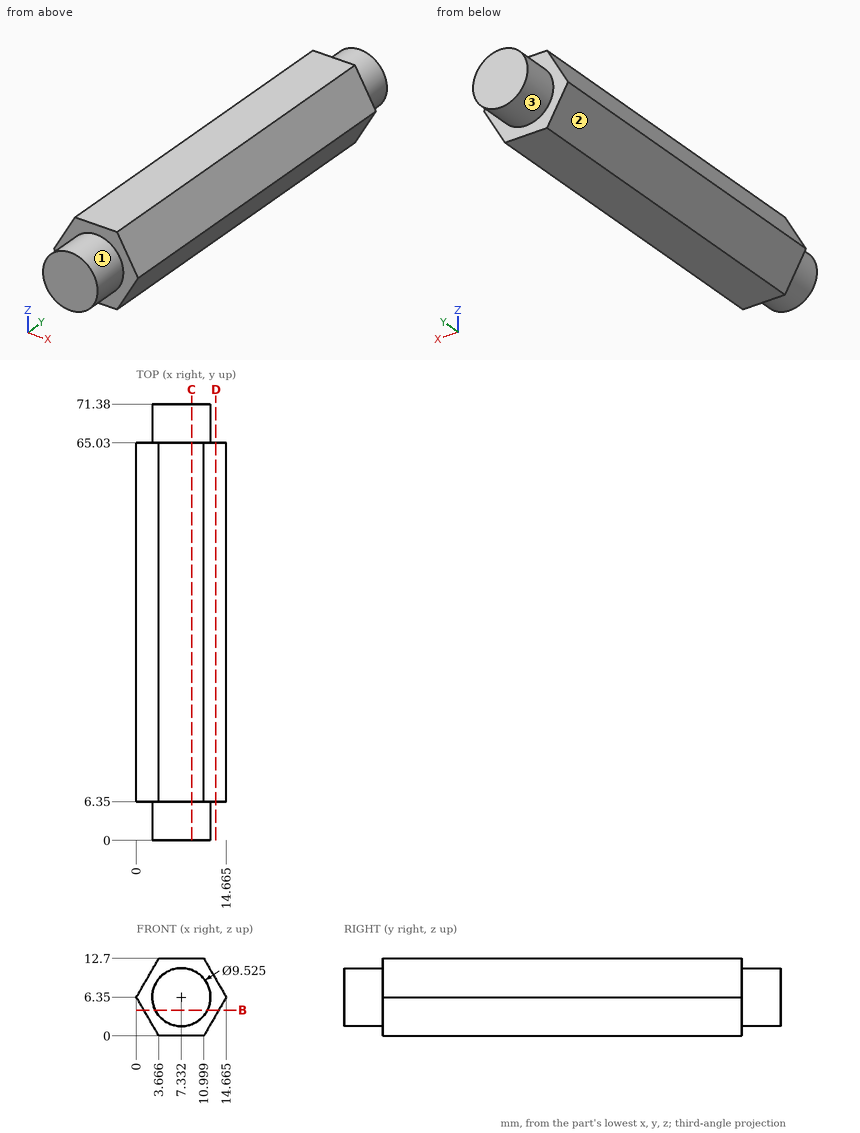
Here's the drawing with two shaded views (mm, measured from the low corner). I have some questions. A direction names the side the tool comes from. Give positions to 0.01 mm unless a question says otherwise; leave off trailing zeros. Loops run counter-clockwise (first coordinate to the right, second up) from the corner with the lowest first, then second, coordinate; pieces in that order, holes last. Notation, with made-up numbers: (21.25, 63) - (77.25, 63) arc R21 cw to (77.25, 82) - close; hole circle Ø7 at (-19.5, -24.5). An arc over 180 degrees is marked (long way). Answer in a Markdown table with one row per item. Add a question column.
Q1. If we section it at C-C (x = 9): List the corners of the cut face in (y, z) for me.
Q2. If we section it at D-D (x = 13): List the corners of the cut face in (y, z) for me.
Q3. Which directions (+Z, -Z, +X, -X, +Y, -Y) give clear straight access to the entire face, cutting with the end or side of a thin tool? Please do the marked faces 1, 2 and 3.
Q4. If we section it at B-B (z = 4.25): List the corners of the cut face in (x, y) for me, plus the area to 3 significant figures.
Q5. Please list where these lines run through material, in increasing order: L1, parallel to Z at x = 11, y = 38 (1 decimal); L2, parallel to Y at x = 8.25, z = 12; L3, parallel to X at y = 40.5, z = 1.5 (1 decimal). Write a range as from..to.
Q6. For pin 1 (1 mm diameter, centred on x = 10, z = 1.5, fed in from -Y); pin 2 (4 mm diameter, centred on y = 58, z = 10, fed in from +X), each with a flat end and sliding along its axis, tell me the tip position at first contact or that it passes through.
The answers:
| question | item | result |
|---|---|---|
| 1 | outline | (0, 1.89) - (6.35, 1.89) - (6.35, 0) - (65.03, 0) - (65.03, 1.89) - (71.38, 1.89) - (71.38, 10.81) - (65.03, 10.81) - (65.03, 12.7) - (6.35, 12.7) - (6.35, 10.81) - (0, 10.81) - close |
| 2 | outline | (6.35, 3.47) - (65.03, 3.47) - (65.03, 9.23) - (6.35, 9.23) - close |
| 3 | face 1 | -Y |
| 3 | face 2 | -Z, -X, +Y, -Y |
| 3 | face 3 | +Y |
| 4 | outline | (1.21, 6.35) - (3.06, 6.35) - (3.06, 0) - (11.61, 0) - (11.61, 6.35) - (13.45, 6.35) - (13.45, 65.03) - (11.61, 65.03) - (11.61, 71.38) - (3.06, 71.38) - (3.06, 65.03) - (1.21, 65.03) - close |
| 4 | area | 827 mm^2 |
| 5 | L1 | z = 0..12.7 |
| 5 | L2 | y = 6.35..65.03 |
| 5 | L3 | x = 2.8..11.9 |
| 6 | pin 1 | stops at y = 6.35 |
| 6 | pin 2 | stops at x = 13.71 |
